Model file for the job. Use its own axes, mm. Face numbers are marked on the shaded views. A direction names the side the tool comes from. Give positions to 0.01 mm unless a question says otherwise; leave off trailing zeros. Order: outer loops, then holes, each group sorted by start corner. A loop starts at its lowest first (then second) coordinate and runs counter-clockwise, first axis right, second up. Notation, with made-up numbers: M -31,-38 L -2,-38 A20 cw -2,-4 Z; hole C 78,81.5 d8. An arc over 180 degrees is marked long. Return JSON: item names as keys, results as strings. Group by question number.
1. Wall check: probe 1 along Y at (x, z) = (0, 2.5); probe 2 along Y at (x, z) = (-12.5, 4.5); probe 3 along X at (y, z) = (-15, 2). Give the ranges that are in metal, low to high. Write a range as [from, to].
2. Slice it at A-A on y = 22. List the corners of the cut face in (x, z).
3. Two-plate mould, pull along X, no slides. Class the marked faces 1, 2 and 3: released by +X, released by -X, zero draft, split by the parting line, or undercut.
4. Pin check, flat tips, straight feed: pin 1 (1 mm diameter, centred on x = -15.5, z = 6, fed in from +Y); pin 2 (2 mm diameter, centred on x = -12.5, z = 2.5, fed in from -Y); pin 3 (6 mm diameter, centred on x = 2, y = -19, fed in from -Z). Stop position of each tip, or through.
5. 3-axis set-ups, long thin cutter, end or side, ignore diameter. For the marked faces 4 and 5: which of +Z, -Z, +X, -X, +Y, -Y reach the whole face in a straight line?
6. Slice it at C-C on z = 2.5. List the corners of the cut face in (x, y), then the cut area to 3 significant figures.
7. Slice it at B-B on x = 14.5. List the corners of the cut face in (y, z), then the cut area to 3 significant figures.
8. Slice it at D-D on y = -12. List the corners of the cut face in (x, z), then the cut area to 3 significant figures.
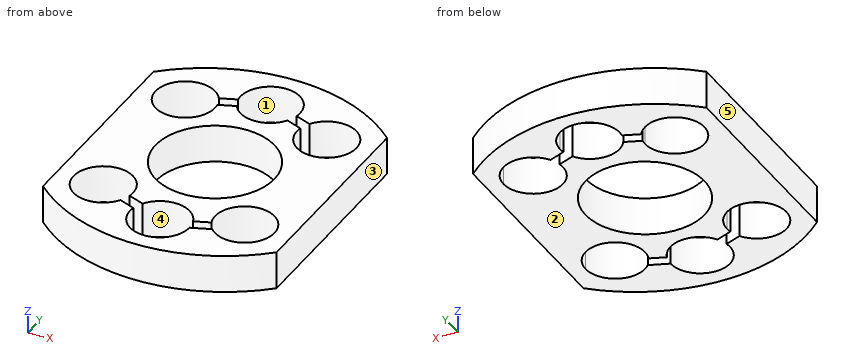
from build123d import *

# Parameters (mm, degrees)
F0_R     = 11
F1_DEPTH = 7


with BuildPart() as f1:
    # F0 (on Top) → F1 (new body)
    with BuildSketch(Plane.XY):
        with BuildLine():
            ThreePointArc((21.529075, 19.597523), (-0.037789, 28.097523), (-21.604652, 19.597523))
            Line((-21.604652, 19.597523), (-21.604652, -19.402477))
            ThreePointArc((-21.604652, -19.402477), (-0.037789, -27.902477), (21.529075, -19.402477))
            Line((21.529075, -19.402477), (21.529075, 19.597523))
        make_face()
        with BuildLine():
            ThreePointArc((-8.415779, -17.251634), (-18.397988, -12.883317), (-7.604652, -14.376836))
            ThreePointArc((-7.604652, -14.376836), (-7.627996, -14.883036), (-7.69783, -15.384939))
            Line((-7.69783, -15.384939), (-4.726662, -16.527678))
            ThreePointArc((-4.726662, -16.527678), (0.464308, -13.925443), (5.095622, -17.428118))
            Line((5.095622, -17.428118), (7.895665, -16.351195))
            ThreePointArc((7.895665, -16.351195), (12.025023, -8.969259), (18.529075, -14.376836))
            ThreePointArc((18.529075, -14.376836), (15.016261, -19.505295), (8.965041, -18.082727))
            Line((8.965041, -18.082727), (5.462211, -19.402477))
            ThreePointArc((5.462211, -19.402477), (-0.543989, -24.879133), (-5.444611, -18.394373))
            Line((-5.444611, -18.394373), (-8.415779, -17.251634))
        make_face(mode=Mode.SUBTRACT)
        with Locations((-0.037789, 0.097523)):
            Circle(F0_R, mode=Mode.SUBTRACT)
        with BuildLine():
            ThreePointArc((8.340202, 17.446681), (14.522594, 19.865218), (18.529075, 14.571882))
            ThreePointArc((18.529075, 14.571882), (12.522875, 9.095226), (7.622253, 15.579986))
            Line((7.622253, 15.579986), (4.651085, 16.722725))
            ThreePointArc((4.651085, 16.722725), (-0.037789, 14.097523), (-4.726662, 16.722725))
            Line((-4.726662, 16.722725), (-7.69783, 15.579986))
            ThreePointArc((-7.69783, 15.579986), (-7.627996, 15.078083), (-7.604652, 14.571882))
            ThreePointArc((-7.604652, 14.571882), (-18.397988, 13.078364), (-8.415779, 17.446681))
            Line((-8.415779, 17.446681), (-5.444611, 18.58942))
            ThreePointArc((-5.444611, 18.58942), (-0.543989, 25.074179), (5.462211, 19.597523))
            ThreePointArc((5.462211, 19.597523), (5.438867, 19.091323), (5.369034, 18.58942))
            Line((5.369034, 18.58942), (8.340202, 17.446681))
        make_face(mode=Mode.SUBTRACT)
    extrude(amount=F1_DEPTH)


solid = f1.part
Result:
{
 "1": {"probe 1": "y = [-27.9, -24.9], [-13.9, -10.9], [11.1, 14.1], [25.1, 28.1]", "probe 2": "y = [-25.34, -19.84], [-8.91, 9.11], [20.04, 25.54]", "probe 3": "x = [-21.6, -18.57], [-7.64, -3.33], [3.26, 7.56], [18.49, 21.53]"},
 "2": {"outline": "M -18.7,0 L -4.99,0 L -4.99,7 L -18.7,7 Z; M 4.91,0 L 18.63,0 L 18.63,7 L 4.91,7 Z"},
 "3": {"face 1": "undercut", "face 2": "zero draft", "face 3": "released by +X"},
 "4": {"pin 1": "stops at y = 24.33", "pin 2": "stops at y = -25.75", "pin 3": "passes through"},
 "5": {"face 4": "+Z, -Z", "face 5": "+Z, -Z, -X, +Y, -Y"},
 "6": {"outline": "M -21.6,-19.4 A31.61 ccw 21.53,-19.4 L 21.53,19.6 A31.61 ccw -21.6,19.6 Z; hole C -0.04,0.1 d22; hole M -8.42,-17.25 L -5.44,-18.39 A5.5 ccw long 5.46,-19.4 L 8.97,-18.08 A5.5 ccw 18.53,-14.38 A5.5 ccw long 7.9,-16.35 L 5.1,-17.43 A5.5 ccw -4.73,-16.53 L -7.7,-15.38 A5.5 ccw -7.6,-14.38 A5.5 ccw long Z; hole M -8.42,17.45 A5.5 ccw long -7.6,14.57 A5.5 ccw -7.7,15.58 L -4.73,16.72 A5.5 ccw 4.65,16.72 L 7.62,15.58 A5.5 ccw long 8.34,17.45 L 5.37,18.59 A5.5 ccw 5.46,19.6 A5.5 ccw long -5.44,18.59 Z", "area": "1,210 mm2"},
 "7": {"outline": "M -24.36,0 L -19.68,0 L -19.68,7 L -24.36,7 Z; M -9.08,0 L 9.27,0 L 9.27,7 L -9.08,7 Z; M 19.87,0 L 24.56,0 L 24.56,7 L 19.87,7 Z", "area": "194 mm2"},
 "8": {"outline": "M -21.6,0 L -18.06,0 L -18.06,7 L -21.6,7 Z; M -8.14,0 L 8.07,0 L 8.07,7 L -8.14,7 Z; M 17.99,0 L 21.53,0 L 21.53,7 L 17.99,7 Z", "area": "163 mm2"}
}
